Geometry check sheet. Reference: drawing and pictorial views, mm from the part's lowest x, y, z. A direction names the side the tool comes from. Round coordinates to 2 decimals unless told otherwise and drop trailing zeros. Loops run counter-clockwise (first coordinate to the right, second up) from the corner with the lowest first, then second, coordinate; pieces in that order, holes last. Notation, with made-up numbers: (3.25, 12.25) - (48.25, 12.25) arc R15 ccw to (48.25, 37.25) - close; hole circle Ø3 at (-18.5, 51). An arc over 180 degrees is marked (long way). Answer in a Markdown table with one row per item. Add a question column.
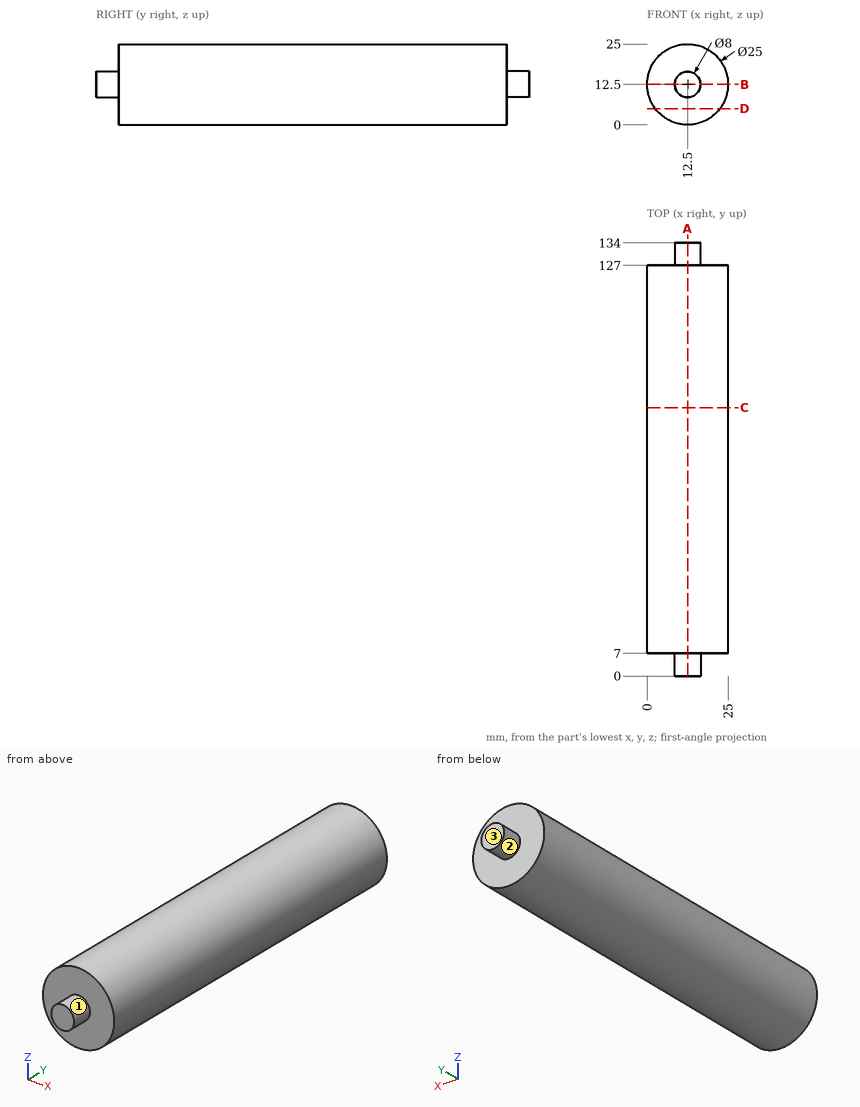
Q1. Depth check by flat-ended pin: P1, Ø5, axis at x = 20, z = 18, coming from the -Y side; P2, Ø1.5, axis at y = 113.5, z = 10, coming from the -X side; P3, Ø8, axis at y = 120.5, z = 3.5, coming from the -X side. Enter the tip coordinate at first touch or a pass-through.
Q2. Cross-section at C-C, the plane y = 83. Enter the section's corners in (x, z), plus the area to 3 significant figures.
Q3. Cross-section at A-A, the plane x = 12.5. Enter the section's corners in (y, z), plus the area to 3 significant figures.
Q4. Cross-section at D-D, the plane z = 5. Enter the section's corners in (x, y).
Q5. Set-up check for the marked faces 1, 2 and 3: record each of +Z, -Z, +X, -X, +Y, -Y from which the full face is reachable in a straight line by a thin tool's end or side.
Q6. Scan lines: line 1 (Z direction, x = 13.25, y = 97); line 2 (Y direction, x = 19.25, z = 17.75); line 3 (Z direction, x = 5.25, y = 23.5). Record each from-to range of solid material in increasing order. Write a range as from..to.
Q7. Cross-section at B-B, the plane z = 12.5. Enter the section's corners in (x, y).
Check sheet entries:
| question | item | result |
|---|---|---|
| 1 | P1 | y = 7 |
| 1 | P2 | x = 0.12 |
| 1 | P3 | x = 1.04 |
| 2 | outline | circle Ø25 at (12.5, 12.5) |
| 2 | area | 491 mm² |
| 3 | outline | (0, 8.5) - (7, 8.5) - (7, 0) - (127, 0) - (127, 8.5) - (134, 8.5) - (134, 16.5) - (127, 16.5) - (127, 25) - (7, 25) - (7, 16.5) - (0, 16.5) - close |
| 3 | area | 3,110 mm² |
| 4 | outline | (2.5, 7) - (22.5, 7) - (22.5, 127) - (2.5, 127) - close |
| 5 | face 1 | -Y |
| 5 | face 2 | +Y |
| 5 | face 3 | +Z, -Z, +X, -X, +Y |
| 6 | line 1 | 0.02..24.98 |
| 6 | line 2 | 7..127 |
| 6 | line 3 | 2.32..22.68 |
| 7 | outline | (0, 7) - (8.5, 7) - (8.5, 0) - (16.5, 0) - (16.5, 7) - (25, 7) - (25, 127) - (16.5, 127) - (16.5, 134) - (8.5, 134) - (8.5, 127) - (0, 127) - close |
